```python
from build123d import *

# Parameters (mm, degrees)
F1_DEPTH    = 2
F2_DEPTH    = 25
F4_DEPTH    = 8
F5_DEPTH    = 4.5
F6_T1_DEPTH = 8
F7_DEPTH    = 3
F8_R        = 2.54
F9_SIZE     = 2.54


# Not quite as in the source:
# - a fillet or chamfer that OpenCascade refuses, or shapes differently, is made with other operations: its cross-section is extruded or revolved along the edge and cut away or added


with BuildPart() as f1:
    # F0 (on Top) → F1 (new body)
    with BuildSketch(Plane.XY):
        with BuildLine():
            Line((6.25, 0), (10, 0))
            ThreePointArc((10, 0), (0, 10), (-10, 0))
            Line((-10, 0), (-6.25, 0))
            ThreePointArc((-6.25, 0), (0, 6.25), (6.25, 0))
        make_face()
    extrude(amount=F1_DEPTH)

    # F0 (on Top) → F2 (join)
    with BuildSketch(Plane.XY):
        with BuildLine():
            ThreePointArc((-10, 0), (0, 10), (10, 0))
            Line((10, 0), (15, 0))
            ThreePointArc((15, 0), (0, 15), (-15, 0))
            Line((-15, 0), (-10, 0))
        make_face()
    extrude(amount=F2_DEPTH)

    # F3 (on face) → F4 (join)
    with BuildSketch(Plane.XY.offset(25)):
        with BuildLine():
            ThreePointArc((-8.75, 12.183492931), (-4.5960638613, 14.2785222268), (0, 15))
            Line((0, 15), (0, 26.25))
            ThreePointArc((0, 26.25), (-6.1871843354, 28.8128156646), (-8.75, 35))
            Line((-8.75, 35), (-8.75, 12.183492931))
        make_face()
        with BuildLine():
            Line((0, 26.25), (0, 15))
            ThreePointArc((0, 15), (4.5960638613, 14.2785222268), (8.75, 12.183492931))
            Line((8.75, 12.183492931), (8.75, 35))
            ThreePointArc((8.75, 35), (6.1871843354, 28.8128156646), (0, 26.25))
        make_face()
        with BuildLine():
            ThreePointArc((8.75, 35), (0, 43.75), (-8.75, 35))
            Line((-8.75, 35), (-3.75, 35))
            ThreePointArc((-3.75, 35), (0, 38.75), (3.75, 35))
            Line((3.75, 35), (8.75, 35))
        make_face()
        with BuildLine():
            Line((8.75, 12.183492931), (8.75, 4.8412291828))
            ThreePointArc((8.75, 4.8412291828), (9.6824583655, 2.5), (10, 0))
            Line((10, 0), (15, 0))
            ThreePointArc((15, 0), (13.346347815, 6.8465319688), (8.75, 12.183492931))
        make_face()
        with BuildLine():
            ThreePointArc((-10, 0), (-9.6824583655, 2.5), (-8.75, 4.8412291828))
            Line((-8.75, 4.8412291828), (-8.75, 12.183492931))
            ThreePointArc((-8.75, 12.183492931), (-13.346347815, 6.8465319688), (-15, 0))
            Line((-15, 0), (-10, 0))
        make_face()
        with BuildLine():
            Line((0, 15), (0, 10))
            ThreePointArc((0, 10), (5.0787650158, 8.6142989218), (8.75, 4.8412291828))
            Line((8.75, 4.8412291828), (8.75, 12.183492931))
            ThreePointArc((8.75, 12.183492931), (4.5960638613, 14.2785222268), (0, 15))
        make_face()
        with BuildLine():
            ThreePointArc((-8.75, 4.8412291828), (-5.0787650158, 8.6142989218), (0, 10))
            Line((0, 10), (0, 15))
            ThreePointArc((0, 15), (-4.5960638613, 14.2785222268), (-8.75, 12.183492931))
            Line((-8.75, 12.183492931), (-8.75, 4.8412291828))
        make_face()
        with BuildLine():
            ThreePointArc((-8.75, 35), (-6.1871843354, 28.8128156646), (0, 26.25))
            Line((0, 26.25), (0, 31.25))
            ThreePointArc((0, 31.25), (-2.6516504294, 32.3483495706), (-3.75, 35))
            Line((-3.75, 35), (-8.75, 35))
        make_face()
        with BuildLine():
            Line((0, 31.25), (0, 26.25))
            ThreePointArc((0, 26.25), (6.1871843354, 28.8128156646), (8.75, 35))
            Line((8.75, 35), (3.75, 35))
            ThreePointArc((3.75, 35), (2.6516504294, 32.3483495706), (0, 31.25))
        make_face()
    extrude(amount=F4_DEPTH)

    # F3 (on face) → F5 (join)
    with BuildSketch(Plane.XY.offset(25)):
        with BuildLine():
            ThreePointArc((3.75, 35), (0, 38.75), (-3.75, 35))
            Line((-3.75, 35), (-2.25, 35))
            ThreePointArc((-2.25, 35), (0, 37.25), (2.25, 35))
            Line((2.25, 35), (3.75, 35))
        make_face()
        with BuildLine():
            ThreePointArc((-3.75, 35), (-2.6516504294, 32.3483495706), (0, 31.25))
            Line((0, 31.25), (0, 32.75))
            ThreePointArc((0, 32.75), (-1.5909902577, 33.4090097423), (-2.25, 35))
            Line((-2.25, 35), (-3.75, 35))
        make_face()
        with BuildLine():
            Line((0, 32.75), (0, 31.25))
            ThreePointArc((0, 31.25), (2.6516504294, 32.3483495706), (3.75, 35))
            Line((3.75, 35), (2.25, 35))
            ThreePointArc((2.25, 35), (1.5909902577, 33.4090097423), (0, 32.75))
        make_face()
    extrude(amount=F5_DEPTH)

    # F6: fillet of radius 5.08 on 2 edges, made by hand

    # F6_s2 → F6_t1 (join)
    with BuildSketch(Plane.XY.offset(25)):
        with BuildLine():
            ThreePointArc((-10.3311752988, 10.8750548019), (-9.1620009917, 12.5540311317), (-8.75, 14.5580733615))
            Line((-8.75, 14.5580733615), (-8.75, 12.183492931))
            ThreePointArc((-8.75, 12.183492931), (-9.5629919628, 11.5563482433), (-10.3311752988, 10.8750548019))
        make_face()
        with BuildLine():
            ThreePointArc((10.3311752988, 10.8750548019), (9.1620009917, 12.5540311317), (8.75, 14.5580733615))
            Line((8.75, 14.5580733615), (8.75, 12.183492931))
            ThreePointArc((8.75, 12.183492931), (9.5629919628, 11.5563482433), (10.3311752988, 10.8750548019))
        make_face()
    extrude(amount=F6_T1_DEPTH)

    # F7 (add): a face of the model
    f7_faces = [f1.faces().sort_by_distance(p)[0] for p in [
        (0, 7.1463690133, 0),
    ]]
    extrude(f7_faces, amount=F7_DEPTH)

    # F8
    f8_edges = [f1.edges().sort_by_distance(p)[0] for p in [
        (0, 15, -3),
    ]]
    fillet(f8_edges, radius=F8_R)

    # F9
    f9_edges = [f1.edges().sort_by_distance(p)[0] for p in [
        (0, 10, 33),
    ]]
    chamfer(f9_edges, length=F9_SIZE)


solid = f1.part
```
Geometry: final body of the model. Coordinates: model frame, mm. A direction names the side the tool comes from. Round coordinates to 2 decimals unless told otherwise and drop trailing zeros. Order: outer loops, then holes, each group sorted by start corner. A loop starts at its lowest first (then second) coordinate and runs counter-clockwise, first axis right, second up. Notation, with made-up numbers: M 2,10.25 L 21,10.25 A21 ccw 21,27.25 Z; hole C 10,-30.5 d8. An arc over 180 degrees is marked long. One line per item, written item: value.
(1) Cut plane B-B (y = 36.5). Return the cut outline in (x, z).
Result sheet:
outline: M -8.62,25 L -1.68,25 L -1.68,29.5 L -3.44,29.5 L -3.44,33 L -8.62,33 Z; M 1.68,25 L 8.62,25 L 8.62,33 L 3.44,33 L 3.44,29.5 L 1.68,29.5 Z
(2) Cut plane C-C (y = 25). Return the cut outline in (x, z), and give its area (3 significant figures).
Result sheet:
outline: M -8.75,25 L 8.75,25 L 8.75,33 L -8.75,33 Z
area: 140 mm2
(3) Cut plane D-D (z = 17.5). Return the cut outline in (x, y), and give its area (3 significant figures).
Result sheet:
outline: M -15,0 L -10,0 A10 cw 10,0 L 15,0 A15 ccw Z
area: 196 mm2
(4) Reachability of faces 4 (the flat face through (8.75, 25, 29)), 5 (the flat face through (2, 33, 29.5)), 6 (the cylindrical face through (0, 15, 17)), 7 (the flat face through (-8.75, 25, 29)) from +Z, -Z, +X, -X, +Y, -Y: full face, straight path, thin tool, end or side. Return the list, or none.
Result sheet:
face 4: +Z, -Z, +X, +Y
face 5: +Z
face 6: -Z, +Y
face 7: +Z, -Z, -X, +Y
(5) Pin query (flat end, axial travel): P1, Ø1, axis at x = -6.5, y = 34.5, coming from the -Z side; P2, Ø2.5, axis at y = 27, z = 30, coming from the -X side; P3, Ø4, axis at y = 11.5, z = 25.5, coming from the +X side; P4, Ø10, axis at x = 8, z = 26.5, coming from the -Y side. Return the tip coordinate at first contact, or that it passes through.
Result sheet:
P1: z = 25
P2: x = -8.75
P3: x = 11.61
P4: y = 0
(6) Cut plane A-A (z = 27). Return the cut outline in (x, y).
Result sheet:
outline: M -15,0 L -10,0 A10 cw 10,0 L 15,0 A15 ccw 10.33,10.88 A5.08 cw 8.75,14.56 L 8.75,35 A8.75 ccw -8.75,35 L -8.75,14.56 A5.08 cw -10.33,10.88 A15 ccw Z; hole C 0,35 d4.5
(7) Line query: probe 1 along Z at (x, y) = (5, 32.5); probe 2 along Z at (x, y) = (6, 6.5); probe 3 along X at (y, z) = (3, 1). Output: solid intervals per line, ascending. Write a range as [from, to].
Result sheet:
probe 1: [25, 33]
probe 2: [-3, 2]
probe 3: [-14.7, -5.48], [5.48, 14.7]
(8) Pull-direction query (X, two-part tool) for faces 1 (the flat face through (13, 0, 15)), 2 (the flat face through (0, 7, 2)), 3 (the cylindrical face through (0.192, 43.748, 28.944)); classes: pulls with the +X half, pulls with the -X half, needs draft (parallel to the pull), parting line crosses it, or undercut.
Result sheet:
face 1: needs draft
face 2: undercut
face 3: parting line crosses it
